from build123d import *

# Parameters (mm, degrees)
F0_R     = 74.009235
F1_DEPTH = 81.534
F3_DEPTH = 226.06


with BuildPart() as f1:
    # F0 (on Right) → F1 (new body)
    with BuildSketch(Plane.YZ):
        Circle(F0_R)
    extrude(amount=F1_DEPTH)

    # F2 (on face) → F3 (cut)
    with BuildSketch(Plane.YZ):
        Polygon((54.283541, 4.519317), (12.476411, 53.023261), (-46.572695, 28.250861), (-41.259919, -35.563269), (21.072662, -50.230169), align=None)
    extrude(amount=F3_DEPTH, mode=Mode.SUBTRACT)


solid = f1.part
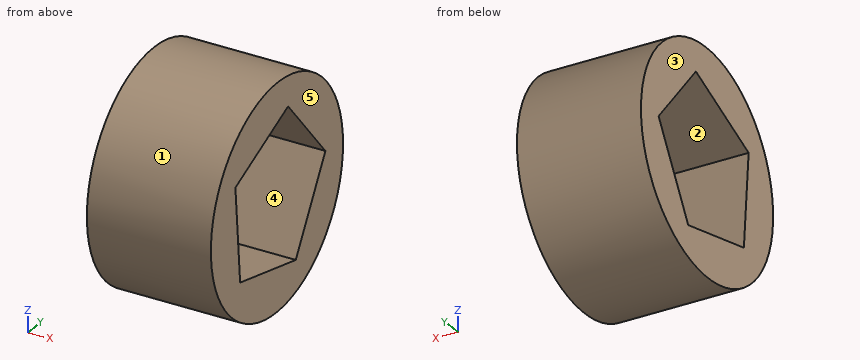
Read the model definition and answer for the solid it produces. Units are mm, in the model's axes. Face numbers are marked on the shaded views. A direction names the side the tool comes from. Coordinates: 2 decimals unless noted, no trailing zeros. Loops run counter-clockwise (first coordinate to the right, second up) from the corner with the lowest first, then second, coordinate; pieces in that order, holes last. Notation, with made-up numbers: (45, 19.5) -> (71, 19.5) arc R31 cw to (71, 53.5) -> close; hole circle Ø3 at (-13, -8.75). An arc over 180 degrees is marked (long way). Write item = value, one per line. Start each with the question number.
1) The mould has two halves that part along Z. Classify the marked faces 1, 2 and 3: pulls with the +Z half, pulls with the -Z half, needs draft (parallel to the pull), parting line crosses it, or undercut.
2) Given P1, Ø1.5, axis at x = 29.5, z = -4.5, coming from the +Y side; P2, Ø10, axis at x = 58.5, z = -22.5, coming from the -Y side; P3, Ø5, axis at x = 51.5, y = -54, coming from the +Z side, each flat-ended and moving along its own axis, determine where each tip first touches the part or whether it passes through.
3) For the marked faces 4 and 5, determine the directions among +Z, -Z, +X, -X, +Y, -Y from which every point of the face is accessible in a straight line to the end or side of a thin tool.
4) The part is cut by section C-C, the plane x = 48.5. Determine the outline of the cut face in (y, z), plus the area to 3 significant figures.
5) The part is cut by section D-D, the plane y = 58.5. Determine the outline of the cut face in (x, z).
6) The part is cut by section B-B, the plane z = 0. Determine the outline of the cut face in (x, y).
7) Find the intervals of material crossed by L1, parallel to Y at x = 32, z = -9; L2, parallel to Z at x = 13, y = -9.5; L3, parallel to Z at x = 21, y = -27, in increasing order. Write a range as from..to.
8) The part is cut by section A-A, the plane y = -10. Determine the outline of the cut face in (x, z), plus the area to 3 significant figures.
Result:
q1.face_1 = parting line crosses it
q1.face_2 = undercut
q1.face_3 = needs draft
q2.P1 = 73.91
q2.P2 = -71.91
q2.P3 = 53.15
q3.face_4 = +X, -X
q3.face_5 = +Z, -Z, +X, +Y, -Y
q4.outline = circle Ø148.02 at (0, 0); hole (-46.57, 28.25) -> (-41.26, -35.56) -> (21.07, -50.23) -> (54.28, 4.52) -> (12.48, 53.02) -> close
q4.area = 10,200 mm²
q5.outline = (0, -45.33) -> (81.53, -45.33) -> (81.53, 45.33) -> (0, 45.33) -> close
q6.outline = (0, -74.01) -> (81.53, -74.01) -> (81.53, -44.22) -> (0, -44.22) -> close; (0, 51.54) -> (81.53, 51.54) -> (81.53, 74.01) -> (0, 74.01) -> close
q7.L1 = -73.46..-43.47, 46.08..73.46
q7.L2 = -73.4..-43.04, 43.8..73.4
q7.L3 = -68.91..-38.92, 36.46..68.91
q8.outline = (0, -73.33) -> (81.53, -73.33) -> (81.53, -42.92) -> (0, -42.92) -> close; (0, 43.59) -> (81.53, 43.59) -> (81.53, 73.33) -> (0, 73.33) -> close
q8.area = 4,900 mm²
